Autodesk Inventor part; units mm, degrees
ref_plane "YZ Plane" through (0, 0, 0) normal (1, 0, 0) x (0, 1, 0)
ref_plane "XZ Plane" through (0, 0, 0) normal (0, 1, 0) x (-1, 0, 0)
ref_plane "XY Plane" through (0, 0, 0) normal (0, 0, 1) x (1, 0, 0)
sketch "Esquisse1" plane through (0, 0, 0) normal (0, 1, 0) x (-1, 0, 0)
  line L0 (0, 0) -> (250, 0)
  line L1 (250, 0) -> (250, -25)
  line L2 (250, -25) -> (0, -25)
  line L3 (0, -25) -> (0, 0)
  line L4 (14.24, 0) -> (14.24, -25) construction
  line L5 (0, -12.5) -> (250, -12.5) construction
  circle A0 centre (14.24, -1.8) radius 1.5
  circle A1 centre (14.24, -23.2) radius 1.5
  circle A2 centre (79.24, -1.8) radius 1.5
  circle A3 centre (79.24, -23.2) radius 1.5
  line L6 (229.7, 0) -> (229.7, -25) construction
  circle A4 centre (229.7, -1.8) radius 1.5
  circle A5 centre (229.7, -23.2) radius 1.5
  circle A6 centre (165, -1.8) radius 1.5
  circle A7 centre (165, -23.2) radius 1.5
  dimension "d0" = 25
  dimension "d1" = 250
  dimension "d2" = 1.8
  dimension "d3" = 3
  dimension "d4" = 14.24
  dimension "d7" = 65
  dimension "d12" = 3
  dimension "d13" = 1.8
  dimension "d17" = 64.7
  dimension "d32" = 165
extrude "Extrusion1" add sketch "Esquisse1" along normal blind 1.6
sketch "Esquisse2" plane through (0, 1.6, 0) normal (0, 1, 0) x (1, 0, 0)
  circle A0 centre (-165, 23.2) radius 1.5 construction
  circle A1 centre (-165, 1.8) radius 1.5 construction
  circle A2 centre (-229.7, 23.2) radius 1.5 construction
  circle A3 centre (-229.7, 1.8) radius 1.5 construction
  circle A4 centre (-79.24, 1.8) radius 1.5 construction
  circle A5 centre (-79.24, 23.2) radius 1.5 construction
  circle A6 centre (-14.24, 23.2) radius 1.5 construction
  circle A7 centre (-14.24, 1.8) radius 1.5 construction
  line L0 (-250, 0) -> (0, 0) construction
  line L1 (0, 0) -> (0, 25) construction
  line L2 (0, 25) -> (-250, 25) construction
  line L3 (-250, 25) -> (-250, 0) construction
  line L4 (-250, 8) -> (-236, 8)
  line L5 (-236, 8) -> (-236, 20)
  line L6 (-236, 20) -> (-250, 20)
  line L7 (-250, 20) -> (-250, 8)
  line L8 (-250, 14) -> (-236, 14) construction
  dimension "d24" = 14
  dimension "d25" = 14
  dimension "d26" = 12
extrude "Extrusion2" add sketch "Esquisse2" along normal blind 7
sketch "Esquisse3" plane through (-250, 0, -25) normal (-1, 0, 0) x (0, 0, 1)
  line L0 (25, 0) -> (0, 0)
  line L1 (25, 0) -> (25, 1.6)
  line L2 (17, 1.6) -> (25, 1.6)
  line L3 (17, 1.6) -> (17, 8.6)
  line L4 (5, 6.6) -> (17, 6.6)
  line L5 (5, 1.6) -> (5, 8.6)
  line L6 (0, 1.6) -> (5, 1.6)
  line L7 (0, 0) -> (0, 1.6)
  line L8 (5, 8.6) -> (17, 8.6) construction
  line L9 (11, 6.6) -> (11, 0) construction
  circle A0 centre (11, 4.1) radius 1.25
  dimension "d29" = 2.5
equation "\"d12\" = d3"
equation "\"d13\" = d2"
properties part number "electronics"
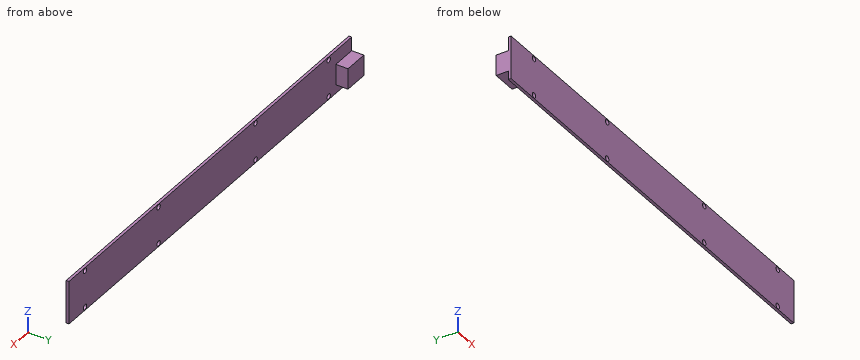
Source: CAD feature listing. Evaluate the final solid. Frame: model axes, mm. Round coordinates to 2 decimals unless told otherwise and drop trailing zeros. Write each loop counter-clockwise with the first axis right and the second up, starting at its lowest first coordinate (ties: lowest second). Pieces come first, ordered by that corner, then holes. Notation, with made-up numbers: M 41,62 L 88,62 A36 cw 88,97 Z; hole C -17.75,-8 d7. An arc over 180 degrees is marked long. Answer as a JSON object with one key per item and string values. Group by question number.
(1) Section query A-A on z = -15.5. Output: boundary loops of the cut face in (x, y).
(2) Section query B-B on y = 5.5. Output: boundary loops of the cut face in (x, z), then the cut area to 3 significant figures.
(3) First-contact query: pin 1 (4 mm diameter, centred on x = -14.24, z = -23.2, fed in from -Y); pin 2 (2 mm diameter, centred on y = 4.5, z = -16, fed in from +X); pin 3 (3.5 mm diameter, centred on x = -240, y = 6.5, fed in from -Z); pin 4 (5 mm diameter, centred on x = -14.24, z = -1.8, fed in from +Y). Flat tips, straight axial feed; report the tip coordinate or a pass-through.
(4) Ray query, line 1 (Z direction, x = -165, y = 0.9); line 2 (Y direction, x = -219, z = -16); line 3 (X direction, y = 2, z = -13.75). Return the intervals inside material, ascending. Write a range as [from, to].
(5) Section query C-C on x = -119. Output: boundary loops of the cut face in (y, z), then the cut area to 3 significant figures.
Computed values:
{
 "1": {"outline": "M -250,0 L 0,0 L 0,1.6 L -236,1.6 L -236,8.6 L -250,8.6 Z"},
 "2": {"outline": "M -250,-20 L -236,-20 L -236,-8 L -250,-8 Z", "area": "168 mm^2"},
 "3": {"pin 1": "y = 0", "pin 2": "x = -236", "pin 3": "z = -20", "pin 4": "y = 1.6"},
 "4": {"line 1": "[-25, -24.7], [-21.7, -3.3], [-0.3, 0]", "line 2": "[0, 1.6]", "line 3": "[-250, -236]"},
 "5": {"outline": "M 0,-25 L 1.6,-25 L 1.6,0 L 0,0 Z", "area": "40.0 mm^2"}
}
